Source: three-view drawing plus pictorial views. Frame: mm from the lowest corner of the part. A direction names the side the tool comes from. Give positions to 0.01 mm unless a question says otherwise; leave off trailing zeros. Order: outer loops, then holes, each group sorted by start corner. A loop starts at its lowest first (then second) coordinate and runs counter-clockwise, first axis right, second up. Notation, with made-up numbers: M -28,59.5 L -12,59.5 A21 cw -12,93.5 Z; hole C -35,41.25 d1. An arc over 180 degrees is marked long. Use CSV: the item, a comma, the result in double quotes. Start each with the question number.
Item 1: Access query for the marked faces 1 and 2. Directions: +Z, -Z, +X, -X, +Y, -Y. A direction counts if a zero-diameter tool reaches every point of the face in a straight line with its end or side. Return the directions, or none.
Item 2: Ray query, probe 1 along X at (y, z) = (3.1, 14); probe 2 along X at (y, z) = (2.6, 4); probe 3 along X at (y, z) = (0.6, 18.25). Return the intervals inside material, ascending. Write a range as from..to.
Item 3: Section query C-C on y = 0.8. Return loops of the section in (x, z), and give its area (3 significant figures).
Item 4: Section query B-B on x = 5. Return loops of the section in (y, z).
Item 5: Section query D-D on z = 4. Return loops of the section in (x, y), and give its area (3 significant figures).
Item 6: Section query A-A on z = 8.5. Return loops of the section in (x, y).
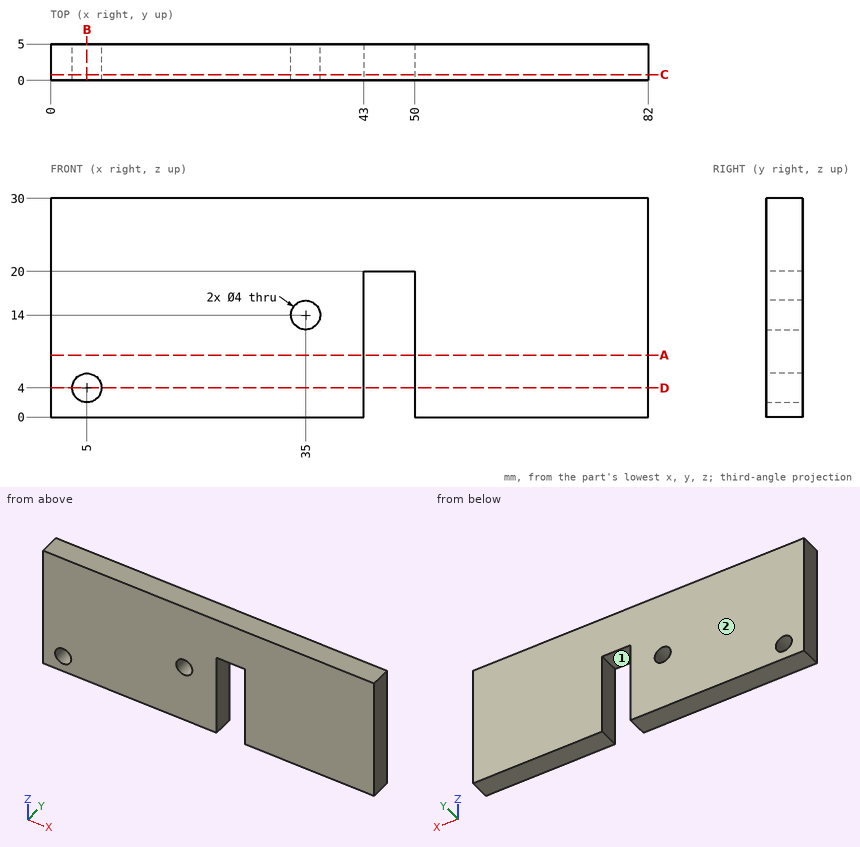
Verdict:
1,face 1,"-Z, +Y, -Y"
1,face 2,"+Z, -Z, +X, -X, +Y"
2,probe 1,"0..33, 37..43, 50..82"
2,probe 2,"0..3, 7..43, 50..82"
2,probe 3,"0..43, 50..82"
3,outline,"M 0,0 L 43,0 L 43,20 L 50,20 L 50,0 L 82,0 L 82,30 L 0,30 Z; hole C 5,4 d4; hole C 35,14 d4"
3,area,"2,290 mm2"
4,outline,"M 0,0 L 5,0 L 5,2 L 0,2 Z; M 0,6 L 5,6 L 5,30 L 0,30 Z"
5,outline,"M 0,0 L 3,0 L 3,5 L 0,5 Z; M 7,0 L 43,0 L 43,5 L 7,5 Z; M 50,0 L 82,0 L 82,5 L 50,5 Z"
5,area,"355 mm2"
6,outline,"M 0,0 L 43,0 L 43,5 L 0,5 Z; M 50,0 L 82,0 L 82,5 L 50,5 Z"
